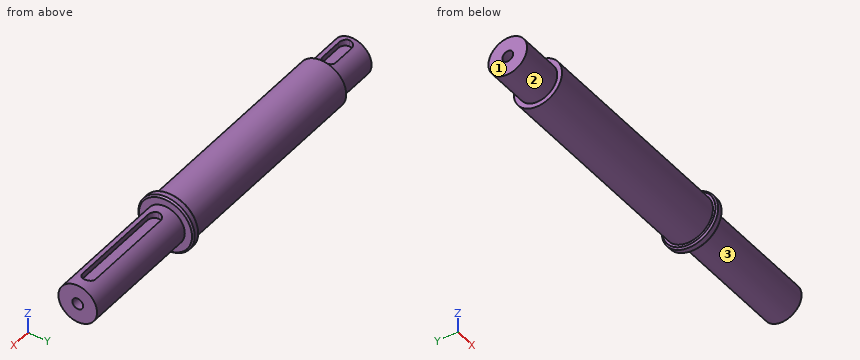
```python
from build123d import *

# Parameters (mm, degrees)
F0_R      = 15
F1_DEPTH  = 164
F2_R      = 12
F3_DEPTH  = 77
F5_D      = 6.8
F5_DEPTH  = 30
F5_TIP    = 2.0429261047
F8_DEPTH  = 4.1
F9_R      = 17.5
F9_R_2    = 15
F10_DEPTH = 5
F11_SIZE  = 1
F12_R     = 15
F12_R_2   = 12
F13_DEPTH = 26.5
F14_D     = 6.8
F14_DEPTH = 20.75
F14_TIP   = 2.0429261047
F16_DEPTH = 4.1


# Not quite as in the source:
# - a feature names something its author has since deleted; it is built from what else it names


with BuildPart() as f1:
    # F0 (on Right) → F1 (new body)
    with BuildSketch(Plane.YZ):
        Circle(F0_R)
    extrude(amount=F1_DEPTH)

    # F2 (on face) → F3 (join)
    with BuildSketch(Plane.YZ.offset(164)):
        Circle(F2_R)
    extrude(amount=F3_DEPTH)

    # F5
    with Locations(Plane.YZ.offset(241)):
        with Locations((0, 0)):
            Hole(F5_D / 2, depth=F5_DEPTH)
            with Locations((0, 0, -(F5_DEPTH + F5_TIP / 2))):  # 118° drill point
                Cone(0, F5_D / 2, F5_TIP, mode=Mode.SUBTRACT)

    # F7 (on offset) → F8 (cut)
    with BuildSketch(Plane.XY.offset(12)):
        with BuildLine():
            ThreePointArc((170, 0), (171.1715728753, -2.8284271247), (174, -4))
            Line((174, -4), (231, -4))
            ThreePointArc((231, -4), (233.8284271247, -2.8284271247), (235, 0))
            ThreePointArc((235, 0), (233.8284271247, 2.8284271247), (231, 4))
            Line((231, 4), (174, 4))
            ThreePointArc((174, 4), (171.1715728753, 2.8284271247), (170, 0))
        make_face()
    extrude(amount=-F8_DEPTH, mode=Mode.SUBTRACT)

    # F9 (on face) → F10 (join)
    with BuildSketch(Plane.YZ.offset(164)):
        Circle(F9_R)
        Circle(F9_R_2, mode=Mode.SUBTRACT)
    extrude(amount=-F10_DEPTH)

    # F11
    f11_edges = [f1.edges().sort_by_distance(p)[0] for p in [
        (164, -17.5, 0),
        (159, -17.5, 0),
    ]]
    chamfer(f11_edges, length=F11_SIZE)

    # F12 (on face) → F13 (cut)
    with BuildSketch(Plane(origin=(0, 0, 0), x_dir=(0, -1, 0), z_dir=(-1, 0, 0))):
        Circle(F12_R)
        Circle(F12_R_2, mode=Mode.SUBTRACT)
    extrude(amount=-F13_DEPTH, mode=Mode.SUBTRACT)

    # F14
    with Locations(Plane(origin=(0, 0, 0), x_dir=(0, -1, 0), z_dir=(-1, 0, 0))):
        with Locations((0, 0)):
            Hole(F14_D / 2, depth=F14_DEPTH)
            with Locations((0, 0, -(F14_DEPTH + F14_TIP / 2))):  # 118° drill point
                Cone(0, F14_D / 2, F14_TIP, mode=Mode.SUBTRACT)

    # F15 (on offset) → F16 (cut)
    with BuildSketch(Plane.XY.offset(12)):
        with BuildLine():
            Line((6.25, -4), (20.25, -4))
            ThreePointArc((20.25, -4), (23.0784271247, -2.8284271247), (24.25, 0))
            ThreePointArc((24.25, 0), (23.0784271247, 2.8284271247), (20.25, 4))
            Line((20.25, 4), (6.25, 4))
            ThreePointArc((6.25, 4), (3.4215728753, 2.8284271247), (2.25, 0))
            ThreePointArc((2.25, 0), (3.4215728753, -2.8284271247), (6.25, -4))
        make_face()
    extrude(amount=-F16_DEPTH, mode=Mode.SUBTRACT)


solid = f1.part
```
Design review of the part built by this model. Coordinates are the model's own, in mm. Face numbers are marked on the shaded views. A direction names the side the tool comes from. Coordinates: 2 decimals unless noted, no trailing zeros. Write each loop counter-clockwise with the first axis right and the second up, starting at its lowest first coordinate (ties: lowest second). Pieces come first, ordered by that corner, then holes.
1) Add section B-B (x = 127). Write out the cut boundary in (y, z).
2) Insertion check: pin 1 (4 mm diameter, centred on y = 0, z = 0, fed in from +X); pin 2 (10 mm diameter, centred on x = 143.5, y = 9, fed in from +Z); pin 3 (12 mm diameter, centred on y = 1.5, z = 2.5, fed in from -X); pin 4 (4 mm diameter, centred on x = 101, y = 6, fed in from -Z). Each pin has a flat end and moves straight along its axis. Give the tip position at first contact, or say it passes through.
3) Machinability: for the marked faces 1, 2 and 3, which of the approach directions +Z, -Z, +X, -X, +Y, -Y give a long, thin tool a straight path to every point of the face, cutting with its end or side? Answer none if there is none.
4) Add section A-A (x = 223.5). Write out the cut boundary in (y, z), plus the area to 3 significant figures.
5) To check wall thickness, follow L1, parallel to Z at x = 227, y = 0; L2, parallel to X at y = -12.5, z = 9; L3, parallel to X at y = 5.5, z = -13.5. State the ranges of each line that lie inside material, in increasing order.
6) Add section C-C (x = 197.5). Write out the cut boundary in (y, z), plus the area to 3 significant figures.
Check result:
1. outline: circle Ø30 at (0, 0)
2. pin 1: stops at x = 210.16
2. pin 2: stops at z = 14.46
2. pin 3: stops at x = 0
2. pin 4: stops at z = -14.46
3. face 1: +Z, -Z, -X, +Y, -Y
3. face 2: -X
3. face 3: +X
4. outline: (-4, 7.9) - (-4, 11.31) arc R12 ccw (long way) to (4, 11.31) - (4, 7.9) - close; hole circle Ø6.8 at (0, 0)
4. area: 385 mm2
5. L1: z = -12 to -3.4, 3.4 to 7.9
5. L2: x = 159 to 164
5. L3: x = 26.5 to 164
6. outline: (-4, 7.9) - (-4, 11.31) arc R12 ccw (long way) to (4, 11.31) - (4, 7.9) - close
6. area: 421 mm2
